Could you check a few things on this drawing? It's one solid part, dimensions in mm from its lowest x, y, z. Round coordinates to 2 decimals unless told otherwise and drop trailing zeros. Write each loop counter-clockwise with the first axis right and the second up, starting at its lowest first coordinate (ties: lowest second). Pieces come first, ordered by that corner, then holes. Notation, with made-up numbers: (42.25, 54.5) - (79.25, 54.5) arc R21 cw to (79.25, 64.5) - close; hole circle Ø8 at (60.25, 48). An arc over 180 degrees is marked (long way). Put each result on its own line as item: value.
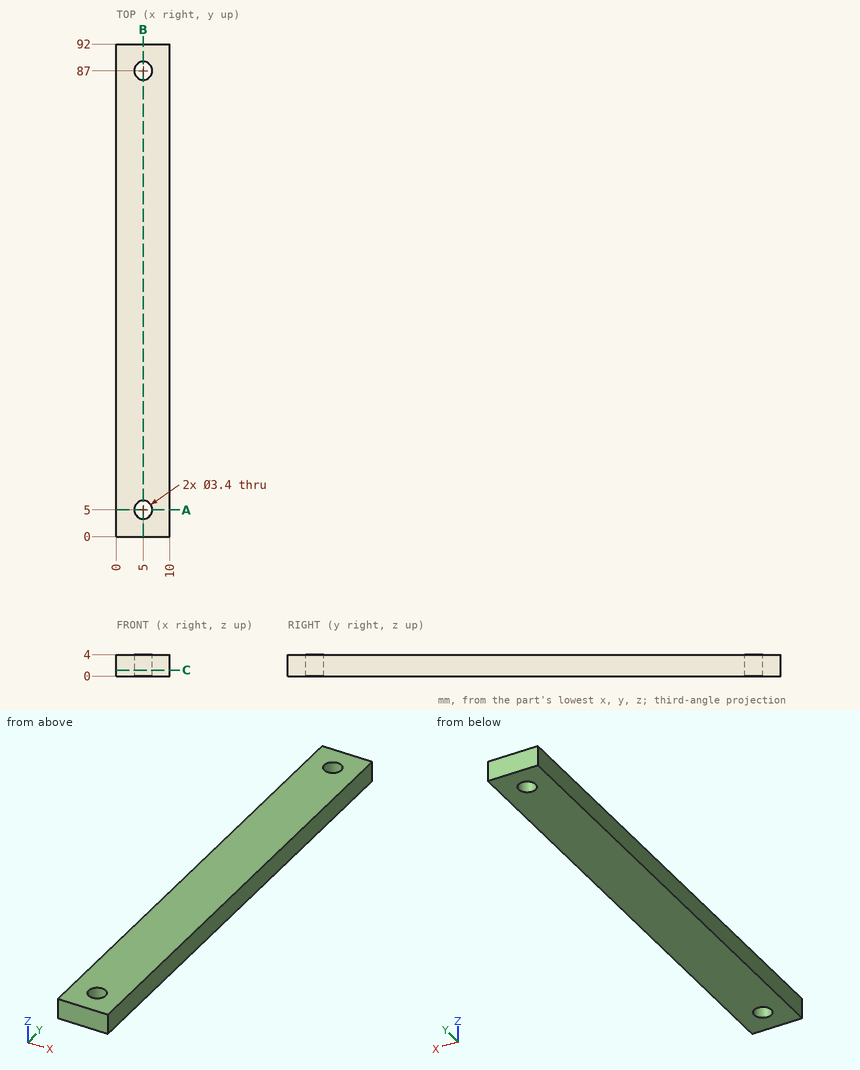
(1) Imagine slicing it at B-B, the plane x = 5. List the corners of the cut face in (y, z) for me, then the cut area to 3 significant figures.
Values found:
outline: (0, 0) - (3.3, 0) - (3.3, 4) - (0, 4) - close; (6.7, 0) - (85.3, 0) - (85.3, 4) - (6.7, 4) - close; (88.7, 0) - (92, 0) - (92, 4) - (88.7, 4) - close
area: 341 mm^2
(2) I'm going to push flat-ended pins straight in: pin 1 (1.5 mm diameter, centred on x = 9, z = 0.5, fed in from -Y); pin 2 (2.5 mm diameter, centred on x = 5, y = 5, fed in from -Z). Where does each tip first touch, or does it pass through?
Values found:
pin 1: stops at y = 0
pin 2: passes through
(3) Please list where these lines run through material, in increasing order: probe 1 along Y at (x, z) = (5, 1.6); probe 2 along Y at (x, z) = (6, 3.85); probe 3 along X at (y, z) = (5, 2.5). Write a range as from..to.
Values found:
probe 1: y = 0..3.3, 6.7..85.3, 88.7..92
probe 2: y = 0..3.63, 6.37..85.63, 88.37..92
probe 3: x = 0..3.3, 6.7..10
(4) Imagine slicing it at A-A, the plane y = 5. List the corners of the cut face in (x, z) for me.
Values found:
outline: (0, 0) - (3.3, 0) - (3.3, 4) - (0, 4) - close; (6.7, 0) - (10, 0) - (10, 4) - (6.7, 4) - close
(5) Imagine slicing it at C-C, the plane z = 1.1. List the corners of the cut face in (x, y) for me, then the cut area to 3 significant figures.
Values found:
outline: (0, 0) - (10, 0) - (10, 92) - (0, 92) - close; hole circle Ø3.4 at (5, 5); hole circle Ø3.4 at (5, 87)
area: 902 mm^2
